Input: part model. Units: mm. Frame: model coordinates. A direction names the side the tool comes from. Coordinates: 2 decimals unless noted, no trailing zeros. Order: outer loops, then holes, each group sorted by start corner. A loop starts at its lowest first (then second) coordinate and runs counter-clockwise, first axis right, second up.
from build123d import *

# Parameters (mm, degrees)
F0_R     = 25.4
F1_DEPTH = 6.35
F3_DEPTH = 12.7
F5_COUNT = 6


with BuildPart() as f1:
    # F0 (on Front) → F1 (new body, symmetric)
    with BuildSketch(Plane.XZ):
        Circle(F0_R)
    extrude(amount=F1_DEPTH, both=True)

    # F2 (on face) → F3 (join)
    with BuildSketch(Plane(origin=(0, 6.35, 0), x_dir=(-1, 0, 0), z_dir=(0, 1, 0))):
        Polygon((0, -24.534516), (0, 0), (-6.574004, -24.534516), align=None)
        Polygon((6.574004, -24.534516), (0, 0), (0, -24.534516), align=None)
        Polygon((6.574004, -34.694516), (6.574004, -24.534516), (0, -24.534516), (-6.574004, -24.534516), (-6.574004, -34.694516), align=None)
        with BuildLine():
            Line((-6.574004, -24.534516), (0, 0))
            Line((0, 0), (6.574004, -24.534516))
            ThreePointArc((6.574004, -24.534516), (20.151175, -15.46254), (25.4, 0))
            ThreePointArc((25.4, 0), (-15.46254, 20.151175), (-6.574004, -24.534516))
        make_face()
    extrude(amount=-F3_DEPTH)

    # F5: F1 ×6 about axis
    f5_axis = Axis((0, -24.47786, 0), (0, -1, 0))


with BuildPart() as f1_1:
    add(f1.part)
    for i in range(1, F5_COUNT):
        add(f1.part.rotate(f5_axis, i * 360 / F5_COUNT))


solid = f1_1.part
Item 1: Ray query, probe 1 along X at (y, z) = (2.5, -6.5); probe 2 along X at (y, z) = (-5.25, 30); probe 3 along Z at (x, y) = (27.5, 2.5). Return the intervals inside material, ascending.
Response values:
probe 1: x = -24.55 to 24.55
probe 2: x = -6.57 to 6.57
probe 3: z = -21.76 to -8.29, 8.29 to 21.76
Item 2: Cut plane A-A on y = -0.5. Return loops of the section in (x, z), then the cut area to 3 significant figures.
Response values:
outline: (-33.33, -11.65) - (-26.76, -23.04) - (-17.96, -17.96) arc R25.4 ccw to (-6.57, -24.53) - (-6.57, -34.69) - (6.57, -34.69) - (6.57, -24.53) arc R25.4 ccw to (17.96, -17.96) - (26.76, -23.04) - (33.33, -11.65) - (24.53, -6.57) arc R25.4 ccw to (24.53, 6.57) - (33.33, 11.65) - (26.76, 23.04) - (17.96, 17.96) arc R25.4 ccw to (6.57, 24.53) - (6.57, 34.69) - (-6.57, 34.69) - (-6.57, 24.53) arc R25.4 ccw to (-17.96, 17.96) - (-26.76, 23.04) - (-33.33, 11.65) - (-24.53, 6.57) arc R25.4 ccw to (-24.53, -6.57) - close
area: 2,780 mm2
Item 3: Pin query (flat end, axial travel): pin 1 Ø1 at (x, y) = (-19, -2) entering from -Z; pin 2 Ø5 at (y, z) = (0.5, -18) entering from -X; pin 3 Ø2 at (x, y) = (8, 4) entering from +Z. Return the tip coordinate at first contact, or that it passes through.
Response values:
pin 1: stops at z = -18.85
pin 2: stops at x = -31.11
pin 3: stops at z = 24.42
Item 4: Cut plane C-C on z = -29. Return loops of the section in (x, y).
Response values:
outline: (-6.57, -6.35) - (6.57, -6.35) - (6.57, 6.35) - (-6.57, 6.35) - close
Item 5: Draft query along X for faces 6 (the face through (6.574, 0, 30)), 7 (the face through (-28.872, 0.089, 9.078)), 8 (the face through (12.78, -0.09, 21.95)). Return one class per face: pulls with the +X half, pulls with the -X half, needs draft (parallel to the pull), parting line crosses it, or undercut.
Response values:
face 6: pulls with the +X half
face 7: pulls with the -X half
face 8: undercut
Item 6: Cut plane B-B on x = 28. Return loops of the section in (y, z), then the cut area to 3 significant figures.
Response values:
outline: (-6.35, -20.89) - (6.35, -20.89) - (6.35, -8.57) - (-6.35, -8.57) - close; (-6.35, 8.57) - (6.35, 8.57) - (6.35, 20.89) - (-6.35, 20.89) - close
area: 313 mm2
Item 7: Access query for faces 1 (the face through (-29, 0.09, -9.15)), 2 (the face through (-6.574, 0, 30)), 3 (the face through (-22.422, 0.089, 20.536)), 4 (the face through (-6.574, 0, -30)), 5 (the face through (22.422, 0.089, -20.536)). Directions: +Z, -Z, +X, -X, +Y, -Y. A direction counts if a zero-diameter tool reaches every point of the face in a straight line with its end or side. Return the directions, or none.
Response values:
face 1: -X, +Y, -Y
face 2: +Z, -X, +Y, -Y
face 3: +Z, +Y, -Y
face 4: -Z, -X, +Y, -Y
face 5: -Z, +Y, -Y
Item 8: Cut plane D-D on x = -20. Return loops of the section in (y, z), then the cut area to 3 significant figures.
Response values:
outline: (-6.35, -19.14) - (6.35, -19.14) - (6.35, 19.14) - (-6.35, 19.14) - close
area: 486 mm2
